Source: CAD feature listing. Evaluate the final solid. Frame: model axes, mm. Face numbers are marked on the shaded views. A direction names the side the tool comes from. Round coordinates to 2 decimals unless told otherwise and drop trailing zeros. Loops run counter-clockwise (first coordinate to the right, second up) from the corner with the lowest first, then second, coordinate; pieces in that order, holes last. Notation, with made-up numbers: (-30, 86) -> (5, 86) arc R27 cw to (5, 110) -> close; hole circle Ø5 at (17, 20.5). An arc over 180 degrees is marked (long way). Put each result on its own line as item: value. Start each with the question number.
1. Cut plane B-B (x = 14.5). Return the cut outline in (y, z).
2. Cut plane D-D (x = -44). Return the cut outline in (y, z), then the cut area to 3 significant figures.
3. Cut plane C-C (z = 6). Return the cut outline in (x, y).
4. Set-up query: the marked faces 1, 2 and 3. Return all of +Z, -Z, +X, -X, +Y, -Y with unobstructed straight access to the full face (end or side cutting, diameter ignored); none if empty.
5. Contact query for flat-ended pins moving along their axis: pin 1 (2 mm diameter, centred on y = -4.5, z = 6, fed in from -X); pin 2 (1 mm diameter, centred on y = -9, z = 5.5, fed in from +X); pin 3 (6.5 mm diameter, centred on x = 14.5, y = -9, fed in from +Z); pin 4 (3 mm diameter, centred on x = -14.5, y = -9, fed in from +Z). Output: stop coordinate, or through.
6. Material intervals for L1, parallel to X at y = -14.5, z = 2; L2, parallel to Y at x = -44, z = 2.5; L3, parallel to X at y = -15.5, z = 0.75, sorted ascending.
7. Draft query along X for the marked faces 4 and 5. Return one class per face: pulls with the +X half, pulls with the -X half, needs draft (parallel to the pull), parting line crosses it, or undercut.
8. Cut plane A-A (y = -9). Return the cut outline in (x, z).
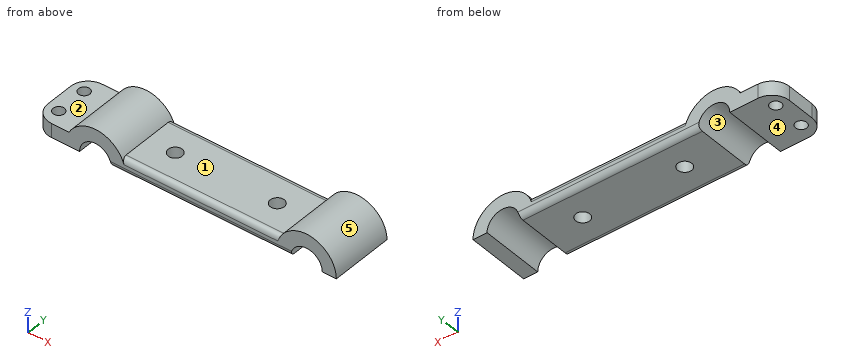
```python
from build123d import *

# Parameters (mm, degrees)
F1_DEPTH = 18
F2_R     = 5
F3_R     = 1.5
F4_R     = 1.6
F5_DEPTH = 4
F4_R_2   = 2
F6_DEPTH = 4


with BuildPart() as f1:
    # F0 (on Front) → F1 (new body)
    with BuildSketch(Plane.XZ):
        with BuildLine():
            ThreePointArc((25.5, 0), (30, 4.5), (34.5, 0))
            Line((34.5, 0), (38.5, 0))
            ThreePointArc((38.5, 0), (32.061553, 8.246211), (22.5, 4))
            Line((22.5, 4), (-22.5, 4))
            ThreePointArc((-22.5, 4), (-30, 8.5), (-37.5, 4))
            Line((-37.5, 4), (-44.5, 4))
            Line((-44.5, 4), (-47.5, 4))
            Line((-47.5, 4), (-47.5, 0))
            Line((-47.5, 0), (-38.5, 0))
            Line((-38.5, 0), (-34.5, 0))
            ThreePointArc((-34.5, 0), (-30, 4.5), (-25.5, 0))
            Line((-25.5, 0), (25.5, 0))
        make_face()
    extrude(amount=F1_DEPTH)

    # F2
    f2_edges = [f1.edges().sort_by_distance(p)[0] for p in [
        (-47.5, -18, 2),
        (-47.5, 0, 2),
    ]]
    fillet(f2_edges, radius=F2_R)

    # F3
    f3_edges = [f1.edges().sort_by_distance(p)[0] for p in [
        (0, -18, 4),
        (0, -18, 0),
        (0, 0, 4),
        (0, 0, 0),
    ]]
    fillet(f3_edges, radius=F3_R)

    # F4 (on face) → F5 (cut, through all)
    with BuildSketch(Plane.XY.offset(4)):
        with Locations((-44, -4.5)):
            Circle(F4_R)
        with Locations((-44, -13.5)):
            Circle(F4_R)
    extrude(amount=-F5_DEPTH, mode=Mode.SUBTRACT)

    # F4 (on face) → F6 (cut, through all)
    with BuildSketch(Plane.XY.offset(4)):
        with Locations((14.5, -9)):
            Circle(F4_R_2)
        with Locations((-14.5, -9)):
            Circle(F4_R_2)
    extrude(amount=-F6_DEPTH, mode=Mode.SUBTRACT)


solid = f1.part
```
Solution:
1. outline: (-18, 1.5) arc R1.5 ccw to (-16.5, 0) -> (-11, 0) -> (-11, 4) -> (-16.5, 4) arc R1.5 ccw to (-18, 2.5) -> close; (-7, 0) -> (-1.5, 0) arc R1.5 ccw to (0, 1.5) -> (0, 2.5) arc R1.5 ccw to (-1.5, 4) -> (-7, 4) -> close
2. outline: (-17.77, 0) -> (-15.1, 0) -> (-15.1, 4) -> (-17.77, 4) -> close; (-11.9, 0) -> (-6.1, 0) -> (-6.1, 4) -> (-11.9, 4) -> close; (-2.9, 0) -> (-0.23, 0) -> (-0.23, 4) -> (-2.9, 4) -> close
2. area: 44.6 mm^2
3. outline: (-36.02, -18) -> (-23.98, -18) -> (-23.98, 0) -> (-36.02, 0) -> close; (23.98, -18) -> (36.02, -18) -> (36.02, 0) -> (23.98, 0) -> close
4. face 1: +Z, +Y, -Y
4. face 2: +Z, -X, +Y, -Y
4. face 3: -Z, +Y, -Y
5. pin 1: stops at x = -36.87
5. pin 2: stops at x = 36.87
5. pin 3: stops at z = 4
5. pin 4: passes through
6. L1: x = -47.27 to -45.25, -42.75 to -34.03, -25.97 to 25.97, 34.03 to 38.26
6. L2: y = -17.77 to -15.1, -11.9 to -6.1, -2.9 to -0.23
6. L3: x = -46.83 to -34.44, -25.56 to 25.56, 34.44 to 38.47
7. face 4: needs draft
7. face 5: undercut
8. outline: (-47.5, 0) -> (-34.5, 0) arc R4.5 cw to (-25.5, 0) -> (-16.5, 0) -> (-16.5, 4) -> (-22.5, 4) arc R8.5 ccw to (-37.5, 4) -> (-47.5, 4) -> close; (-12.5, 0) -> (12.5, 0) -> (12.5, 4) -> (-12.5, 4) -> close; (16.5, 0) -> (25.5, 0) arc R4.5 cw to (34.5, 0) -> (38.5, 0) arc R8.5 ccw to (22.5, 4) -> (16.5, 4) -> close
